```python
from build123d import *

# Parameters (mm, degrees)
F0_W     = 42.3
F0_H     = 42.3
F1_DEPTH = 39
F2_R     = 11
F3_DEPTH = 2
F4_R     = 2.5
F5_DEPTH = 24
F6_SIZE  = 2.5
F8_D     = 2.4
F8_DEPTH = 12
F8_TIP   = 0.7210327428


with BuildPart() as f1:
    # F0 (on Top) → F1 (new body)
    with BuildSketch(Plane.XY):
        with Locations((21.15, 21.15)):
            Rectangle(F0_W, F0_H)
    extrude(amount=F1_DEPTH)

    # F2 (on face) → F3 (join)
    with BuildSketch(Plane.XY.offset(39)):
        with Locations((21.15, 21.15)):
            Circle(F2_R)
    extrude(amount=F3_DEPTH)

    # F4 (on face) → F5 (join)
    with BuildSketch(Plane.XY.offset(41)):
        with Locations((21.15, 21.15)):
            Circle(F4_R)
    extrude(amount=F5_DEPTH)

    # F6
    f6_edges = [f1.edges().sort_by_distance(p)[0] for p in [
        (42.3, 0, 19.5),
        (42.3, 42.3, 19.5),
        (0, 0, 19.5),
        (0, 42.3, 19.5),
    ]]
    chamfer(f6_edges, length=F6_SIZE)

    # F8
    with Locations(Plane.XY.offset(39)):
        with Locations((5.65, 36.65), (36.65, 36.65), (36.65, 5.65), (5.65, 5.65)):
            Hole(F8_D / 2, depth=F8_DEPTH)
            with Locations((0, 0, -(F8_DEPTH + F8_TIP / 2))):  # 118° drill point
                Cone(0, F8_D / 2, F8_TIP, mode=Mode.SUBTRACT)


solid = f1.part
```
CAD build for the part. Positions are in the model's coordinates, mm. A direction names the side the tool comes from. Round coordinates to 2 decimals unless told otherwise and drop trailing zeros. Order: outer loops, then holes, each group sorted by start corner. A loop starts at its lowest first (then second) coordinate and runs counter-clockwise, first axis right, second up.
Q1. Which spindle directions (+Z, -Z, +X, -X, +Y, -Y) get a long thin tool onto all of the face, cutting with end or side? Do faces 5 (the flat face through (21, 21, 0)), 6 (the cylindrical face through (4.54, 5.19, 32.92)). Say none if no direction does.
Q2. Wall check: L1, parallel to X at y = 36.65, z = 33; L2, parallel to Y at x = 5, z = 31. Give the ranges that are in metal, low to high.
Q3. Slice it at A-A (y = 21.15). Write the cut outline in (x, z), and give its area (3 significant figures).
Q4. Drop flat-ended pins along their axis: pin 1 (5 mm diameter, centred on x = 22, y = 26, fed in from -Z); pin 2 (4 mm diameter, centred on y = 18.5, z = 44.5, fed in from -X); pin 3 (2 mm diameter, centred on x = 36.65, y = 5.65, fed in from +Z); pin 4 (3 mm diameter, centred on x = 36.65, y = 36.65, fed in from +Z). Give the stop position or say it passes through.
Q5. Two-plate mould, pull along X, no slides. Class faces 1 (the flat face through (21, 0, 19)), 2 (the cylindrical face through (36.91, 35.48, 32.92)), 3 (the flat face through (41.1, 41, 19.2)), 4 (the conical face through (5.485, 5.523, 26.404)): pulls with the +X half, pulls with the -X half, needs draft (parallel to the pull), parting line crosses it, or undercut.
Q6. Slice it at D-D (x = 11). Write the cut outline in (y, z).
Q7. Slice it at C-C (z = 45). Write the cut outline in (x, y).
Results below:
1. face 5: -Z, +X, -X, +Y, -Y
1. face 6: +Z
2. L1: x = 0 to 4.45, 6.85 to 35.45, 37.85 to 42.3
2. L2: y = 0 to 4.64, 6.66 to 35.64, 37.66 to 42.3
3. outline: (0, 0) - (42.3, 0) - (42.3, 39) - (32.15, 39) - (32.15, 41) - (23.65, 41) - (23.65, 65) - (18.65, 65) - (18.65, 41) - (10.15, 41) - (10.15, 39) - (0, 39) - close
3. area: 1,810 mm2
4. pin 1: stops at z = 0
4. pin 2: stops at x = 18.74
4. pin 3: stops at z = 26.88
4. pin 4: stops at z = 39
5. face 1: needs draft
5. face 2: undercut
5. face 3: pulls with the +X half
5. face 4: undercut
6. outline: (0, 0) - (42.3, 0) - (42.3, 39) - (25.39, 39) - (25.39, 41) - (16.91, 41) - (16.91, 39) - (0, 39) - close
7. outline: circle Ø5 at (21.15, 21.15)
